```python
from build123d import *

# Parameters (mm, degrees)
BOSS_EXTRUDE1_DEPTH = 4.445
SKETCH2_R           = 1.905
SKETCH2_W           = 10.16
SKETCH2_H           = 23.114
BOSS_EXTRUDE2_DEPTH = 2.54
FILLET1_R           = 2.54
SKETCH3_W           = 6.4008
SKETCH3_H           = 64.3636
CUT_EXTRUDE1_DEPTH  = 2.54


with BuildPart() as part:
    # Sketch1 → Boss-Extrude1 (new body)
    with BuildSketch(Plane.XY):
        Polygon((-16.23695, 42.153431645), (-12.63096924, 48.463897975), (12.57381924, 48.463897975), (16.1798, 42.153431645), (16.1798, -42.507635695), (12.57381924, -48.818102025), (-12.63096924, -48.818102025), (-16.23695, -42.507635695), align=None)
        Polygon((-13.69695, 41.478897975), (-11.15695, 45.923897975), (11.0998, 45.923897975), (13.6398, 41.478897975), (13.6398, -41.833102025), (11.0998, -46.278102025), (-11.15695, -46.278102025), (-13.69695, -41.833102025), align=None, mode=Mode.SUBTRACT)
    extrude(amount=BOSS_EXTRUDE1_DEPTH)

    # Sketch2 → Boss-Extrude2 (add)
    with BuildSketch(Plane.XY.offset(4.445)):
        Polygon((-16.23695, 42.153431645), (-16.23695, -42.507635695), (-12.63096924, -48.818102025), (12.57381924, -48.818102025), (16.1798, -42.507635695), (16.1798, 42.153431645), (12.57381924, 48.463897975), (-12.63096924, 48.463897975), align=None)
        with Locations((0, 42.2275)):
            Circle(SKETCH2_R, mode=Mode.SUBTRACT)
        with Locations((0, -42.2275)):
            Circle(SKETCH2_R, mode=Mode.SUBTRACT)
        Rectangle(SKETCH2_W, SKETCH2_H, mode=Mode.SUBTRACT)
    extrude(amount=BOSS_EXTRUDE2_DEPTH)

    # Fillet1
    fillet1_edges = [part.edges().sort_by_distance(p)[0] for p in [
        (-16.23695, 42.153431645, 3.4925),
        (-12.63096924, 48.463897975, 3.4925),
        (12.57381924, 48.463897975, 3.4925),
        (16.1798, 42.153431645, 3.4925),
        (16.1798, -42.507635695, 3.4925),
        (12.57381924, -48.818102025, 3.4925),
        (-12.63096924, -48.818102025, 3.4925),
        (-16.23695, -42.507635695, 3.4925),
        (-14.43395962, 45.30866481, 6.985),
        (-16.23695, -0.177102025, 6.985),
        (-14.43395962, -45.66286886, 6.985),
        (-0.028575, -48.818102025, 6.985),
        (14.37680962, -45.66286886, 6.985),
        (16.1798, -0.177102025, 6.985),
        (14.37680962, 45.30866481, 6.985),
        (-0.028575, 48.463897975, 6.985),
    ]]
    fillet(fillet1_edges, radius=FILLET1_R)

    # Sketch3 → Cut-Extrude1 (cut)
    with BuildSketch(Plane(origin=(16.1798, 0, 0), x_dir=(0, 0, -1), z_dir=(1, 0, 0))):
        Rectangle(SKETCH3_W, SKETCH3_H)
    extrude(amount=-CUT_EXTRUDE1_DEPTH, mode=Mode.SUBTRACT)


solid = part.part
```
The model under review builds one solid part; all positions refer to its coordinate system, in mm. A direction names the side the tool comes from. Round coordinates to 2 decimals unless told otherwise and drop trailing zeros. Loops run counter-clockwise (first coordinate to the right, second up) from the corner with the lowest first, then second, coordinate; pieces in that order, holes last. Notation, with made-up numbers: (22, 0.5) -> (47, 0.5) arc R22 ccw to (47, 28.5) -> close; hole circle Ø1 at (42, 25.25). An arc over 180 degrees is marked (long way). Answer as a JSON object with one key per item and string values. Group by question number.
1) For faces 4 (the face through (0, -11.557, 6)), 5 (the face through (12.4, -44, 2.2)), 6 (the face through (-12.416, 48.13, 2.191)), list the 3-axis set-ups (+Z, -Z, +X, -X, +Y, -Y) from which the entire face can be reached by the end or side of a thin tool; tool diameter is ignored.
2) We need section B-B on x = -7. Write out the cut boundary in (y, z) (3 decimals).
3) We need section C-C on x = 0. Write out the cut boundary in (y, z) (1 decimal), then the cut area to 3 significant figures.
4) Mouldability with a two-part tool opening along Y and no side actions: class faces 1 (the face through (-14.65, -45.285, 2.191)), 2 (the face through (5.08, 0, 6)), 3 (the face through (0, 48.464, 2)) as released by +Y, released by -Y, zero draft, split by the parting line, or undercut.
5) We need section D-D on y = 21. Write out the cut boundary in (x, z) (3 decimals), then the cut area to 3 significant figures.
6) For pin 1 Ø8 at (x, y) = (-0.5, -18.5) entering from -Z (3 decimals); pin 2 Ø1.3 at (x, z) = (15, 2) entering from +Y; pin 3 Ø2 at (y, z) = (21.5, 2) entering from +X; pin 4 Ø5 at (x, y) = (0, 42.23) entering from +Z (3 decimals), all flat-tipped, find the tip position at first contact; note any pin that passes through.
7) For line 1 (X direction, y = 13, z = 3.5); line 2 (Y direction, x = 0, z = 5.45); line 3 (Y direction, x = 0, z = 5.75), list the stretches that pass through material, from the lowest coordinate up. Write a range as [from, to].
8) We need section A-A on y = -5.5. Write out the cut boundary in (x, z) (3 decimals), then the cut area to 3 significant figures.
Result set:
{
 "1": {"face 4": "+Z, -Z", "face 5": "-Z", "face 6": "+Z, -Z, -X, +Y"},
 "2": {"outline": "(-48.818, 0) -> (-46.278, 0) -> (-46.278, 4.445) -> (45.924, 4.445) -> (45.924, 0) -> (48.464, 0) -> (48.464, 4.445) arc R2.54 ccw to (45.924, 6.985) -> (-46.278, 6.985) arc R2.54 ccw to (-48.818, 4.445) -> close"},
 "3": {"outline": "(-48.8, 0) -> (-46.3, 0) -> (-46.3, 4.4) -> (-44.1, 4.4) -> (-44.1, 7) -> (-46.3, 7) arc R2.5 ccw to (-48.8, 4.4) -> close; (-40.3, 4.4) -> (-11.6, 4.4) -> (-11.6, 7) -> (-40.3, 7) -> close; (11.6, 4.4) -> (40.3, 4.4) -> (40.3, 7) -> (11.6, 7) -> close; (44.1, 4.4) -> (45.9, 4.4) -> (45.9, 0) -> (48.5, 0) -> (48.5, 4.4) arc R2.5 ccw to (45.9, 7) -> (44.1, 7) -> close", "area": "189 mm²"},
 "4": {"face 1": "released by -Y", "face 2": "undercut", "face 3": "released by +Y"},
 "5": {"outline": "(-16.237, 0) -> (-13.697, 0) -> (-13.697, 4.445) -> (13.64, 4.445) -> (13.64, 3.2) -> (16.18, 3.2) -> (16.18, 4.445) arc R2.54 ccw to (13.64, 6.985) -> (-13.697, 6.985) arc R2.54 ccw to (-16.237, 4.445) -> close", "area": "94.0 mm²"},
 "6": {"pin 1": "z = 4.445", "pin 2": "y = 45.36", "pin 3": "x = -13.7", "pin 4": "z = 6.985"},
 "7": {"line 1": "[-16.24, -13.7], [13.64, 16.18]", "line 2": "[-48.61, -44.13], [-40.32, -11.56], [11.56, 40.32], [44.13, 48.26]", "line 3": "[-48.46, -44.13], [-40.32, -11.56], [11.56, 40.32], [44.13, 48.1]"},
 "8": {"outline": "(-16.237, 0) -> (-13.697, 0) -> (-13.697, 4.445) -> (-5.08, 4.445) -> (-5.08, 6.985) -> (-13.697, 6.985) arc R2.54 ccw to (-16.237, 4.445) -> close; (5.08, 4.445) -> (13.64, 4.445) -> (13.64, 3.2) -> (16.18, 3.2) -> (16.18, 4.445) arc R2.54 ccw to (13.64, 6.985) -> (5.08, 6.985) -> close", "area": "68.2 mm²"}
}
